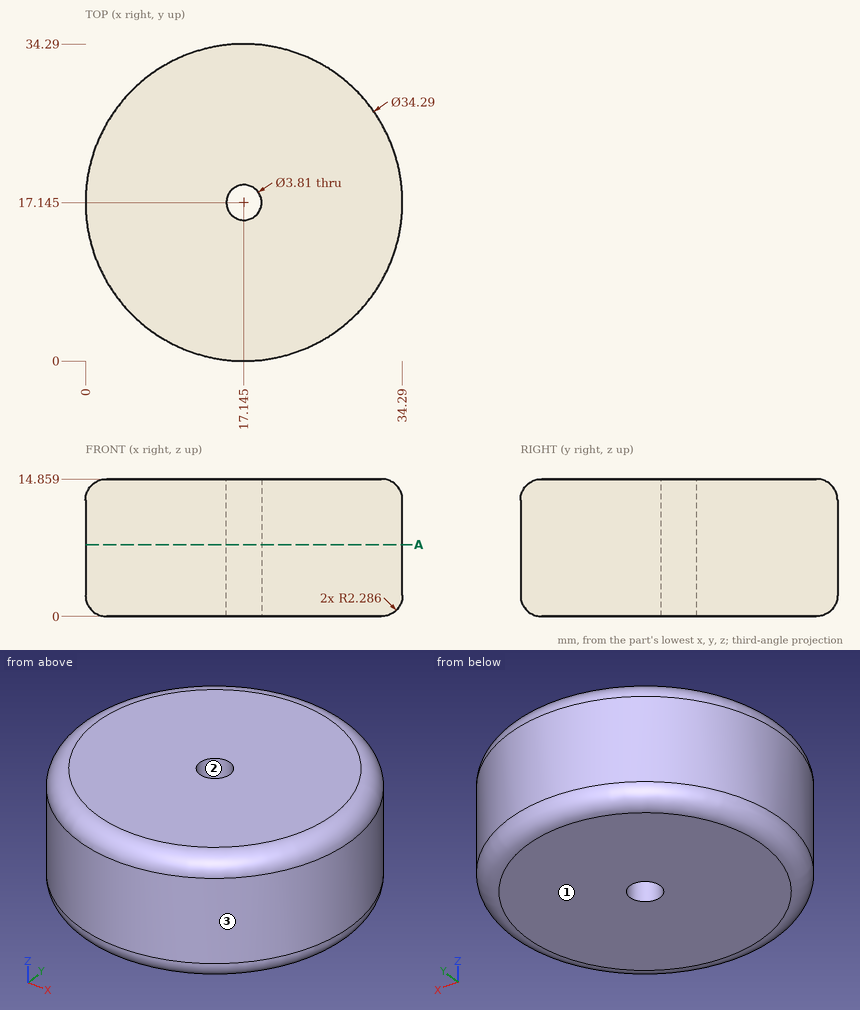
Geometry: see drawing. Coordinates: mm, zero at the bounding-box minimum. Give positions to 0.01 mm unless a question says otherwise; leave off trailing zeros. Loops run counter-clockwise (first coordinate to the right, second up) from the corner with the lowest first, then second, coordinate; pieces in that order, holes last. Notation, with made-up numbers: (-36.75, -26.5) -> (13.25, -26.5) arc R8 cw to (13.25, -16.5) -> close; hole circle Ø2 at (84, 62.5). An arc over 180 degrees is marked (long way). Answer as a JSON object with one key per item and string values. Group by question number.
Item 1: Pin query (flat end, axial travel): P1, Ø1.5, axis at y = 4, z = 6.5, coming from the -X side; P2, Ø4.5, axis at x = 17.145, y = 17.145, coming from the -Z side; P3, Ø8, axis at x = 9.5, z = 6.5, coming from the -Y side; P4, Ø1.5, axis at y = 23, z = 12, coming from the +X side. Return the tip coordinate at first contact, or that it passes through.
Item 2: Line query: probe 1 along Y at (x, z) = (16, 5.25); probe 2 along Y at (x, z) = (30.5, 7.5); probe 3 along X at (y, z) = (28, 6.5). Output: solid intervals per line, ascending.
Item 3: Pull-direction query (X, two-part tool) for the marked faces 1, 2 and 3; classes: released by +X, released by -X, zero draft, split by the parting line, or undercut.
Item 4: Cut plane A-A, the plane z = 7.75. Return the cut outline in (x, y) (3 decimals).
Checks:
{
 "1": {"P1": "stops at x = 5.3", "P2": "stops at z = 0", "P3": "stops at y = 0.39", "P4": "stops at x = 33.51"},
 "2": {"probe 1": "y = 0.04 to 15.62, 18.67 to 34.25", "probe 2": "y = 6.39 to 27.9", "probe 3": "x = 3.87 to 30.42"},
 "3": {"face 1": "zero draft", "face 2": "undercut", "face 3": "split by the parting line"},
 "4": {"outline": "circle Ø34.29 at (17.145, 17.145); hole circle Ø3.81 at (17.145, 17.145)"}
}
